from build123d import *

# Parameters (mm, degrees)
SKETCH1_R             = 2.1
BOSS_EXTRUDE1_DEPTH   = 8
FILLET1_R             = 5
CHAMFER1_SIZE         = 10
CHAMFER1_SIZE2        = 2.867453858
CHAMFER1_PART_2_SIZE  = 10
CHAMFER1_PART_2_SIZE2 = 2.867453858
CUT_EXTRUDE1_REACH    = 10


with BuildPart() as part:
    # Sketch1 → Boss-Extrude1 (new body)
    with BuildSketch(Plane(origin=(0, 0, 0), x_dir=(0, 0, -1), z_dir=(1, 0, 0))):
        with BuildLine():
            Line((10, 30), (-10, 30))
            Line((-10, 30), (-10, 15.850422707))
            ThreePointArc((-10, 15.850422707), (-8.2854567, 8.007496488), (-7.71, 0))
            ThreePointArc((-7.71, 0), (-8.2854567, -8.007496488), (-10, -15.850422707))
            Line((-10, -15.850422707), (-10, -30))
            Line((-10, -30), (10, -30))
            Line((10, -30), (10, 30))
        make_face()
        with Locations((-3.69, -22.685)):
            Circle(SKETCH1_R, mode=Mode.SUBTRACT)
        with Locations((-3.69, 22.685)):
            Circle(SKETCH1_R, mode=Mode.SUBTRACT)
    extrude(amount=-BOSS_EXTRUDE1_DEPTH)

    # Fillet1
    fillet1_edges = [part.edges().sort_by_distance(p)[0] for p in [
        (-4, 30, 10),
        (-4, -30, 10),
    ]]
    fillet(fillet1_edges, radius=FILLET1_R)

    # Chamfer1
    chamfer1_edges = [part.edges().sort_by_distance(p)[0] for p in [
        (-4, 30, -10),
    ]]
    chamfer1_side = [part.faces().sort_by_distance(p)[0] for p in [
        (-4, 30, -2.5),
    ]]
    chamfer(chamfer1_edges, length=CHAMFER1_SIZE, length2=CHAMFER1_SIZE2, reference=chamfer1_side[0])

    # Chamfer1 part 2
    chamfer1_part_2_edges = [part.edges().sort_by_distance(p)[0] for p in [
        (-4, -30, -10),
    ]]
    chamfer1_part_2_side = [part.faces().sort_by_distance(p)[0] for p in [
        (-4, -30, -2.5),
    ]]
    chamfer(chamfer1_part_2_edges, length=CHAMFER1_PART_2_SIZE, length2=CHAMFER1_PART_2_SIZE2, reference=chamfer1_part_2_side[0])

    # Sketch2 → Cut-Extrude1 (cut, up to next)
    with BuildSketch(Plane(origin=(0, 0, 0), x_dir=(0, 0, -1), z_dir=(1, 0, 0)), mode=Mode.PRIVATE) as cut_extrude1_sk1:
        with BuildLine():
            Line((7.725, 16), (7.725, -16))
            ThreePointArc((7.725, -16), (6.225, -17.5), (4.725, -16))
            Line((4.725, -16), (4.725, 16))
            ThreePointArc((4.725, 16), (6.225, 17.5), (7.725, 16))
        make_face()
    cut_extrude1_tool1 = extrude(cut_extrude1_sk1.sketch, amount=-CUT_EXTRUDE1_REACH, mode=Mode.PRIVATE) & part.part
    add(cut_extrude1_tool1.solids().sort_by_distance((0, 0, -6.225))[0], mode=Mode.SUBTRACT)
    # Sketch2 → Cut-Extrude1 (cut, up to next)
    with BuildSketch(Plane(origin=(0, 0, 0), x_dir=(0, 0, -1), z_dir=(1, 0, 0)), mode=Mode.PRIVATE) as cut_extrude1_sk2:
        with BuildLine():
            Line((-5.435, 16), (-5.435, -16))
            ThreePointArc((-5.435, -16), (-3.935, -17.5), (-2.435, -16))
            Line((-2.435, -16), (-2.435, 16))
            ThreePointArc((-2.435, 16), (-3.935, 17.5), (-5.435, 16))
        make_face()
    cut_extrude1_tool2 = extrude(cut_extrude1_sk2.sketch, amount=-CUT_EXTRUDE1_REACH, mode=Mode.PRIVATE) & part.part
    add(cut_extrude1_tool2.solids().sort_by_distance((0, 0, 3.935))[0], mode=Mode.SUBTRACT)


solid = part.part
Input: part model. Units: mm. Frame: model coordinates. A direction names the side the tool comes from. Coordinates: 2 decimals unless noted, no trailing zeros. Loops run counter-clockwise (first coordinate to the right, second up) from the corner with the lowest first, then second, coordinate; pieces in that order, holes last.
(1) Section B-B on x = -7. Return the cut outline in (y, z) (3 decimals), then the cut area to 3 significant figures.
(2) Section A-A on z = -5.75. Return the cut outline in (x, y).
(3) Material intervals for probe 1 along Z at (x, y) = (-3.5, -1) (3 decimals); probe 2 along Z at (x, y) = (-5.5, -12.5) (3 decimals); probe 3 along Y at (x, z) = (-3.5, 2), sorted ascending.
(4) First-contact query: pin 1 Ø3 at (x, z) = (-5.5, -2) entering from +Y. Flat tip, straight axial feed; report the tip coordinate or a pass-through.
(5) Set-up query: faces 5 (the face through (-3.9, 17.5, -6.2)), 6 (the face through (-8, 0, 0)). Return all of +Z, -Z, +X, -X, +Y, -Y with unobstructed straight access to the full face (end or side cutting, diameter ignored); none if empty.
(6) Section C-C on z = -3.25. Return the cut outline in (x, y), then the cut area to 3 significant figures.
(7) Pull-direction query (Z, two-part tool) for faces 1 (the face through (-4, 0, -4.725)), 2 (the face through (-4, 0, -10)), 3 (the face through (-4, -30, 3)), 4 (the face through (-3.9, -17.5, -6.3)); classes: released by +Z, released by -Z, zero draft, split by the parting line, or undercut.
Data:
1. outline: (-30, 0) - (-27.133, -10) - (27.133, -10) - (30, 0) - (30, 5) arc R5 ccw to (25, 10) - (15.85, 10) arc R56 cw to (-15.85, 10) - (-25, 10) arc R5 ccw to (-30, 5) - close; hole circle Ø4.2 at (-22.685, 3.69); hole (-16, -7.725) - (16, -7.725) arc R1.5 ccw to (16, -4.725) - (-16, -4.725) arc R1.5 ccw to start; hole (-16, 2.435) - (16, 2.435) arc R1.5 ccw to (16, 5.435) - (-16, 5.435) arc R1.5 ccw to start; hole circle Ø4.2 at (22.685, 3.69)
1. area: 878 mm2
2. outline: (-8, -28.35) - (0, -28.35) - (0, -17.42) - (-8, -17.42) - close; (-8, 17.42) - (0, 17.42) - (0, 28.35) - (-8, 28.35) - close
3. probe 1: z = -10 to -7.725, -4.725 to 2.435, 5.435 to 7.719
3. probe 2: z = -10 to -7.725, -4.725 to 2.435, 5.435 to 9.123
3. probe 3: y = -30 to -23.93, -21.44 to 21.44, 23.93 to 30
4. pin 1: stops at y = 29.86
5. face 5: +X, -X
5. face 6: +Z, -Z, -X, +Y, -Y
6. outline: (-8, -29.07) - (0, -29.07) - (0, 29.07) - (-8, 29.07) - close
6. area: 465 mm2
7. face 1: undercut
7. face 2: released by -Z
7. face 3: zero draft
7. face 4: undercut
